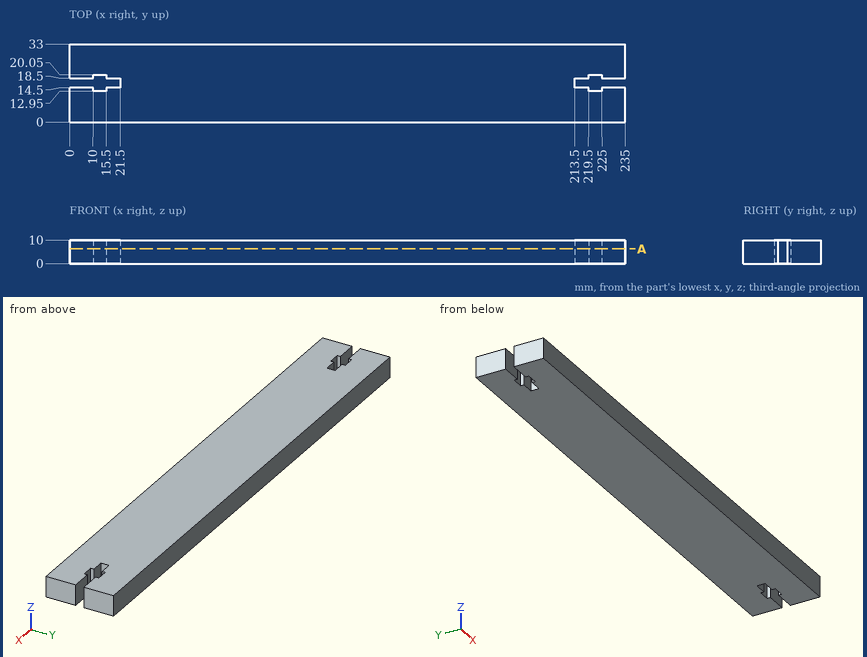
Study the drawing (mm; zero at the part's minimum x, y, z) and answer. Give positions to 0.01 mm unless a question says otherwise; leave off trailing zeros. Loops run counter-clockwise (first coordinate to the right, second up) from the corner with the lowest first, then second, coordinate; pieces in that order, holes last. Notation, with made-up numbers: (12.25, 68.25) -> (58.25, 68.25) arc R7 ccw to (58.25, 75.25) -> close; hole circle Ø3 at (5.5, 88.5). An arc over 180 degrees is marked (long way). Use a Markdown table: item, result. Add a question column.
1) This flat-tipped pin is pushed along its axis until it touches: P1, Ø1.2, axis at y = 16.5, z = 6, coming from the +X side. Where does it stop, or does it pass through?
2) The part is cut by section A-A, the plane z = 6.25. Determine the outline of the cut face in (x, y).
3) Consider line 1 along X through (y, z) = (14, 5.5); line 2 along Y through (x, z) = (215.5, 0.75); line 3 along X through (y, z) = (15.5, 1). Determine where each line is inside the solid, lowest interval first.
Reported:
| question | item | result |
|---|---|---|
| 1 | P1 | stops at x = 213.5 |
| 2 | outline | (0, 0) -> (235, 0) -> (235, 14.5) -> (225, 14.5) -> (225, 12.95) -> (219.5, 12.95) -> (219.5, 14.5) -> (213.5, 14.5) -> (213.5, 18.5) -> (219.5, 18.5) -> (219.5, 20.05) -> (225, 20.05) -> (225, 18.5) -> (235, 18.5) -> (235, 33) -> (0, 33) -> (0, 18.5) -> (10, 18.5) -> (10, 20.05) -> (15.5, 20.05) -> (15.5, 18.5) -> (21.5, 18.5) -> (21.5, 14.5) -> (15.5, 14.5) -> (15.5, 12.95) -> (10, 12.95) -> (10, 14.5) -> (0, 14.5) -> close |
| 3 | line 1 | x = 0 to 10, 15.5 to 219.5, 225 to 235 |
| 3 | line 2 | y = 0 to 14.5, 18.5 to 33 |
| 3 | line 3 | x = 21.5 to 213.5 |
